Could you check a few things on this model? Use its own coordinates, in mm. A direction names the side the tool comes from. Give positions to 0.01 mm unless a question says otherwise; leave off trailing zeros. Order: outer loops, then holes, each group sorted by start corner. A loop starts at its lowest first (then second) coordinate and runs counter-clockwise, first axis right, second up. Notation, with made-up numbers: M -12,-4 L -7,-4 A20 cw -7,27 Z; hole C 77.5,59.25 d3. An arc over 180 degrees is marked long. Use a Markdown table: item, result. Add a question column.
Item 1: For faces 4 (the face through (-29.1, 13, -56)), 5 (the face through (-18, 13, -75)), 6 (the face through (-20.6, 3, 55)), 7 (the face through (-16, 3, -17)), which set-ups out of +Z, -Z, +X, -X, +Y, -Y let a thin tool reach every point of the face, with its end or its side?
Item 2: I'm going to push flat-ended pins straight in: pin 1 Ø3 at (x, z) = (0.5, -11.5) entering from +Y; pin 2 Ø2.5 at (y, z) = (10.94, -59.97) entering from +X; pin 3 Ø2 at (y, z) = (10.94, -59.97) entering from -X; pin 4 Ø8 at (y, z) = (6.87, -56.65) entering from -X. Where does each tip first touch, or does it pass through?
Item 3: If I drill on L1, parallel to Z at x = 13, y = 22.25; L2, parallel to Z at x = 23.5, y = 10.94; L3, parallel to Y at x = -11.5, z = -59.97, over which ranges is the centre line in solid material (lowest first)? Write a range as from..to.
Item 4: If we mould it in two halves opening along Y, with no side actions, what happens to faces 1 (the face through (16, 5.842, -61)), 2 (the face through (-15, 1.75, -69)), 3 (the face through (-2.3, 13, -69))? For each: released by +Y, released by -Y, zero draft, split by the parting line, or undercut.
Item 5: Suppose I cut it at C-C on y = 16. Write out the boundary of the cut face in (x, z).
Item 6: Suppose I cut it at D-D on z = -7. Write out the boundary of the cut face in (x, y).
Item 7: Suppose I cut it at A-A on x = -7.5. Write out the boundary of the cut face in (y, z) (3 decimals), plus the area to 3 significant figures.
Item 8: Suppose I cut it at B-B on z = -38. Write out the boundary of the cut face in (x, y).
from build123d import *

# Parameters (mm, degrees)
SKETCH1_W            = 66.8
SKETCH1_H            = 150
BOSS_EXTRUDE1_DEPTH  = 1.75
SKETCH2_W            = 7
SKETCH2_H            = 12
SKETCH2_W_2          = 2.3
BOSS_EXTRUDE2_DEPTH  = 6
SKETCH3_W            = 19
SKETCH3_H            = 5
BOSS_EXTRUDE3_DEPTH  = 11.79
SKETCH4_R            = 1.1
CUT_EXTRUDE1_DEPTH   = 23.3
SKETCH33_R           = 1.1
BOSS_EXTRUDE21_DEPTH = 1.5
SKETCH8_R            = 8.5
CUT_EXTRUDE3_DEPTH   = 4.3
SKETCH5_W            = 7
SKETCH5_H            = 7.697712298
CUT_EXTRUDE4_DEPTH   = 5
BOSS_EXTRUDE6_DEPTH  = 5
BOSS_EXTRUDE23_DEPTH = 4.3
CUT_EXTRUDE6_REACH   = 92.003
SKETCH36_R           = 3
SKETCH34_W           = 10
SKETCH34_H           = 5
BOSS_EXTRUDE24_DEPTH = 10.61
BOSS_EXTRUDE25_DEPTH = 4.3
BOSS_EXTRUDE26_DEPTH = 5
FILLET7_R            = 1
SKETCH44_W           = 5
SKETCH44_H           = 10.61
BOSS_EXTRUDE30_DEPTH = 14
SKETCH45_W           = 7
SKETCH45_H           = 0.4
CUT_EXTRUDE8_DEPTH   = 5
FILLET7_OF_MIRROR5_R = 1
SKETCH30_R           = 1.1
BOSS_EXTRUDE19_DEPTH = 0.6
SKETCH28_W           = 4.6
SKETCH28_H           = 12
BOSS_EXTRUDE31_DEPTH = 16.4
SKETCH47_W           = 66.8
SKETCH47_H           = 25.9
BOSS_EXTRUDE32_DEPTH = 1.5
SKETCH50_W           = 1.227389953
SKETCH50_H           = 22.4
BOSS_EXTRUDE33_DEPTH = 10.2
CUT_EXTRUDE9_DEPTH   = 2
SKETCH52_W           = 34
SKETCH52_H           = 53
SKETCH52_W_2         = 53
SKETCH52_H_2         = 34
BOSS_EXTRUDE34_DEPTH = 5.7
SKETCH53_W           = 26.2
SKETCH53_H           = 49.2
BOSS_EXTRUDE35_DEPTH = 2.8


# Read off the part's stored shape, not the designer's step: Boss-Extrude6
with BuildPart() as part:
    # Sketch1 → Boss-Extrude1 (new, symmetric)
    with BuildSketch(Plane(origin=(0, 0, 0), x_dir=(1, 0, 0), z_dir=(0, 1, 0))):
        Rectangle(SKETCH1_W, SKETCH1_H)
    boss_extrude1 = extrude(amount=BOSS_EXTRUDE1_DEPTH, both=True)

    # Sketch2 → Boss-Extrude2 (add)
    with BuildSketch(Plane(origin=(0, 1.75, 0), x_dir=(1, 0, 0), z_dir=(0, 1, 0))):
        with Locations((-29.9, 69)):
            Rectangle(SKETCH2_W, SKETCH2_H)
        with Locations((-1.15, 69)):
            Rectangle(SKETCH2_W_2, SKETCH2_H)
    boss_extrude2 = extrude(amount=BOSS_EXTRUDE2_DEPTH)

    # Sketch3 → Boss-Extrude3 (add)
    with BuildSketch(Plane(origin=(0, 1.75, 0), x_dir=(1, 0, 0), z_dir=(0, 1, 0))):
        with Locations((-19.6, 60.5)):
            Rectangle(SKETCH3_W, SKETCH3_H)
    boss_extrude3 = extrude(amount=BOSS_EXTRUDE3_DEPTH)

    # Sketch4 → Cut-Extrude1 (cut)
    with BuildSketch(Plane.ZY.offset(33.4)):
        with Locations((-59.97, 10.94)):
            Circle(SKETCH4_R)
    cut_extrude1 = extrude(amount=-CUT_EXTRUDE1_DEPTH, mode=Mode.SUBTRACT)

    # Sketch33 → Boss-Extrude21 (add)
    with BuildSketch(Plane.ZY.offset(29.1)):
        with BuildLine():
            Line((-58, 1.75), (-32.714619908, 1.75))
            Line((-32.714619908, 1.75), (-32.714619908, 18.755533204))
            ThreePointArc((-32.714619908, 18.755533204), (-32.928979134, 21.486214993), (-33.566805397, 24.15))
            Line((-33.566805397, 24.15), (-58, 24.15))
            Line((-58, 24.15), (-58, 1.75))
        make_face()
        with Locations((-50.214619908, 18.755533204)):
            Circle(SKETCH33_R, mode=Mode.SUBTRACT)
    boss_extrude21 = extrude(amount=-BOSS_EXTRUDE21_DEPTH)

    # Sketch8 → Cut-Extrude3 (cut)
    with BuildSketch(Plane.ZY.offset(29.1)):
        with Locations((-59.97, 10.94)):
            Circle(SKETCH8_R)
    cut_extrude3 = extrude(amount=CUT_EXTRUDE3_DEPTH, mode=Mode.SUBTRACT)

    # Sketch5 → Cut-Extrude4 (cut)
    with BuildSketch(Plane.XY.offset(-58)):
        with Locations((-15.6, 9.691143851)):
            Rectangle(SKETCH5_W, SKETCH5_H)
    cut_extrude4 = extrude(amount=-CUT_EXTRUDE4_DEPTH, mode=Mode.SUBTRACT)

    # Boss-Extrude6 outline → Boss-Extrude6 (add)
    with BuildSketch(Plane(origin=(-10.1, 0, 0), x_dir=(0, 0, -1), z_dir=(1, 0, 0))):
        with BuildLine():
            Line((63, 1.75), (63, 13.54))
            Line((63, 13.54), (58, 13.54))
            Line((58, 13.54), (54.474415859, 12.063241708))
            ThreePointArc((54.474415859, 12.063241708), (51.964403757, 9.99079907), (51.022610047, 6.875))
            Line((51.022610047, 6.875), (51.022610047, 1.75))
            Line((51.022610047, 1.75), (56.647610047, 1.75))
            ThreePointArc((56.647610047, 1.75), (55.965342342, 11.954383405), (58, 1.93165433))
            Line((58, 1.93165433), (58, 1.75))
            Line((58, 1.75), (63, 1.75))
        make_face()
    boss_extrude6 = extrude(amount=BOSS_EXTRUDE6_DEPTH)

    # Sketch35 → Boss-Extrude23 (add)
    with BuildSketch(Plane.ZY.offset(29.1)):
        with BuildLine():
            ThreePointArc((-51.696668378, 12.889867655), (-54.372371702, 4.543394851), (-63, 2.998394369))
            Line((-63, 2.998394369), (-63, 1.75))
            Line((-63, 1.75), (-32.714619908, 1.75))
            Line((-32.714619908, 1.75), (-32.714619908, 18.755533204))
            ThreePointArc((-32.714619908, 18.755533204), (-32.928979134, 21.486214993), (-33.566805397, 24.15))
            Line((-33.566805397, 24.15), (-47.475600378, 24.15))
            ThreePointArc((-47.475600378, 24.15), (-44.549583353, 16.631889912), (-51.696668378, 12.889867655))
        make_face()
        with BuildLine():
            ThreePointArc((-58, 19.208560939), (-57.114293593, 18.945931608), (-56.262320095, 18.588732556))
            ThreePointArc((-56.262320095, 18.588732556), (-55.413998212, 21.848907617), (-52.953639439, 24.15))
            Line((-52.953639439, 24.15), (-58, 24.15))
            Line((-58, 24.15), (-58, 19.208560939))
        make_face()
    boss_extrude23 = extrude(amount=BOSS_EXTRUDE23_DEPTH)

    # Cut-Extrude6: up to this face of the body (flat: up to its plane)
    cut_extrude6_end = Plane(part.part.faces().sort_by_distance((-19.1, 9.554283394, -60.558081983))[0])
    # Sketch36 → Cut-Extrude6 (cut, up to the picked face)
    with BuildSketch(Plane.ZY.offset(10.1), mode=Mode.PRIVATE) as cut_extrude6_sk1:
        with Locations((-56.647610047, 6.875)):
            Circle(SKETCH36_R)
    cut_extrude6_tool1 = split(extrude(cut_extrude6_sk1.sketch, amount=CUT_EXTRUDE6_REACH, mode=Mode.PRIVATE), bisect_by=cut_extrude6_end, keep=Keep.BOTH, mode=Mode.PRIVATE)
    cut_extrude6 = cut_extrude6_tool1.solids().sort_by(Axis((-10.1, 6.875, -56.64761), (-1, 0, 0)))[0]
    add(cut_extrude6, mode=Mode.SUBTRACT)

    # Sketch34 → Boss-Extrude24 (add)
    with BuildSketch(Plane(origin=(0, 13.54, 0), x_dir=(1, 0, 0), z_dir=(0, 1, 0))):
        with Locations((-24.1, 60.5)):
            Rectangle(SKETCH34_W, SKETCH34_H)
    boss_extrude24 = extrude(amount=BOSS_EXTRUDE24_DEPTH)

    # Sketch37 → Boss-Extrude25 (add)
    with BuildSketch(Plane.ZY.offset(29.1)):
        with BuildLine():
            Line((-58, 24.15), (-63, 24.15))
            Line((-63, 24.15), (-63, 18.881605631))
            ThreePointArc((-63, 18.881605631), (-60.524639471, 19.421885112), (-58, 19.208560939))
            Line((-58, 19.208560939), (-58, 24.15))
        make_face()
    boss_extrude25 = extrude(amount=BOSS_EXTRUDE25_DEPTH)

    # Sketch38 → Boss-Extrude26 (add)
    with BuildSketch(Plane.ZY.offset(10.1)):
        with BuildLine():
            Line((-56.647610047, 1.75), (-58.2, 1.75))
            Line((-58.2, 1.75), (-58.2, 1.99076921))
            ThreePointArc((-58.2, 1.99076921), (-57.433085123, 1.810549991), (-56.647610047, 1.75))
        make_face()
    boss_extrude26 = extrude(amount=-BOSS_EXTRUDE26_DEPTH)

    # Fillet7
    fillet7_edges = [part.edges().sort_by_distance(p)[0] for p in [
        (-31.25, 12.889867655, -51.696668378),
        (-31.25, 24.15, -47.475600378),
        (-31.25, 18.588732556, -56.262320095),
        (-31.25, 24.15, -52.953639439),
        (-11.1, 9.552880023, -58),
        (-33.4, 7.75, -71.424349566),
        (-27.75, 7.75, -63),
        (-27.6, 12.95, -58),
    ]]
    fillet(fillet7_edges, radius=FILLET7_R)

    # Sketch44 → Boss-Extrude30 (add)
    with BuildSketch(Plane(origin=(-19.1, 0, 0), x_dir=(0, 0, -1), z_dir=(1, 0, 0))):
        with Locations((60.5, 18.845)):
            Rectangle(SKETCH44_W, SKETCH44_H)
    boss_extrude30 = extrude(amount=BOSS_EXTRUDE30_DEPTH)

    # Sketch45 → Cut-Extrude8 (cut)
    with BuildSketch(Plane.XY.offset(-58)):
        with Locations((-15.6, 13.74)):
            Rectangle(SKETCH45_W, SKETCH45_H)
    cut_extrude8 = extrude(amount=-CUT_EXTRUDE8_DEPTH, mode=Mode.SUBTRACT)

    # Mirror5: Boss-Extrude1, Boss-Extrude2, Boss-Extrude3, Cut-Extrude1, Boss-Extrude21, Cut-Extrude3, Cut-Extrude4, Boss-Extrude6, Boss-Extrude23, Cut-Extrude6, Boss-Extrude24, Boss-Extrude25, Boss-Extrude26, Boss-Extrude30, Cut-Extrude8 across plane
    add(boss_extrude1.mirror(Plane(origin=(0, 0, 0), x_dir=(0, 0, 1), z_dir=(1, 0, 0))))
    add(boss_extrude2.mirror(Plane(origin=(0, 0, 0), x_dir=(0, 0, 1), z_dir=(1, 0, 0))))
    add(boss_extrude3.mirror(Plane(origin=(0, 0, 0), x_dir=(0, 0, 1), z_dir=(1, 0, 0))))
    add(cut_extrude1.mirror(Plane(origin=(0, 0, 0), x_dir=(0, 0, 1), z_dir=(1, 0, 0))), mode=Mode.SUBTRACT)
    add(boss_extrude21.mirror(Plane(origin=(0, 0, 0), x_dir=(0, 0, 1), z_dir=(1, 0, 0))))
    add(cut_extrude3.mirror(Plane(origin=(0, 0, 0), x_dir=(0, 0, 1), z_dir=(1, 0, 0))), mode=Mode.SUBTRACT)
    add(cut_extrude4.mirror(Plane(origin=(0, 0, 0), x_dir=(0, 0, 1), z_dir=(1, 0, 0))), mode=Mode.SUBTRACT)
    add(boss_extrude6.mirror(Plane(origin=(0, 0, 0), x_dir=(0, 0, 1), z_dir=(1, 0, 0))))
    add(boss_extrude23.mirror(Plane(origin=(0, 0, 0), x_dir=(0, 0, 1), z_dir=(1, 0, 0))))
    add(cut_extrude6.mirror(Plane(origin=(0, 0, 0), x_dir=(0, 0, 1), z_dir=(1, 0, 0))), mode=Mode.SUBTRACT)
    add(boss_extrude24.mirror(Plane(origin=(0, 0, 0), x_dir=(0, 0, 1), z_dir=(1, 0, 0))))
    add(boss_extrude25.mirror(Plane(origin=(0, 0, 0), x_dir=(0, 0, 1), z_dir=(1, 0, 0))))
    add(boss_extrude26.mirror(Plane(origin=(0, 0, 0), x_dir=(0, 0, 1), z_dir=(1, 0, 0))))
    add(boss_extrude30.mirror(Plane(origin=(0, 0, 0), x_dir=(0, 0, 1), z_dir=(1, 0, 0))))
    add(cut_extrude8.mirror(Plane(origin=(0, 0, 0), x_dir=(0, 0, 1), z_dir=(1, 0, 0))), mode=Mode.SUBTRACT)

    # Fillet7 of Mirror5
    fillet7_of_mirror5_edges = [part.edges().sort_by_distance(p)[0] for p in [
        (31.25, 12.889867655, -51.696668378),
        (31.25, 24.15, -47.475600378),
        (31.25, 18.588732556, -56.262320095),
        (31.25, 24.15, -52.953639439),
        (11.1, 9.552880023, -58),
        (33.4, 7.75, -71.424349566),
        (27.75, 7.75, -63),
        (27.6, 12.95, -58),
    ]]
    fillet(fillet7_of_mirror5_edges, radius=FILLET7_OF_MIRROR5_R)

    # Sketch30 → Boss-Extrude19 (add)
    with BuildSketch(Plane(origin=(-10.1, 0, 0), x_dir=(0, 0, -1), z_dir=(1, 0, 0))):
        with Locations(Location((59.97, 10.94, 0), (0, 0, 90))):
            Circle(SKETCH30_R)
    boss_extrude19 = extrude(amount=-BOSS_EXTRUDE19_DEPTH)

    # Mirror6: Boss-Extrude19 across plane
    add(boss_extrude19.mirror(Plane(origin=(0, 0, 0), x_dir=(0, 0, 1), z_dir=(1, 0, 0))))

    # Sketch28 → Boss-Extrude31 (add)
    with BuildSketch(Plane(origin=(0, 7.75, 0), x_dir=(1, 0, 0), z_dir=(0, 1, 0))):
        with Locations((0, 69)):
            Rectangle(SKETCH28_W, SKETCH28_H)
    extrude(amount=BOSS_EXTRUDE31_DEPTH)

    # Sketch47 → Boss-Extrude32 (add)
    with BuildSketch(Plane(origin=(0, 0, -75), x_dir=(-1, 0, 0), z_dir=(0, 0, -1))):
        with Locations((0, 11.2)):
            Rectangle(SKETCH47_W, SKETCH47_H)
    extrude(amount=BOSS_EXTRUDE32_DEPTH)

    # Sketch50 → Boss-Extrude33 (add)
    with BuildSketch(Plane.ZY.offset(-5.1)):
        with Locations((-62.386305024, 12.95)):
            Rectangle(SKETCH50_W, SKETCH50_H)
    extrude(amount=BOSS_EXTRUDE33_DEPTH)

    # Sketch51 → Cut-Extrude9 (cut)
    with BuildSketch(Plane(origin=(0, 1.75, 0), x_dir=(1, 0, 0), z_dir=(0, 1, 0))):
        with BuildLine():
            Line((-33.4, 32.714619908), (-33.4, -75))
            Line((-33.4, -75), (33.4, -75))
            Line((33.4, -75), (33.4, 32.714619908))
            Line((33.4, 32.714619908), (27.6, 32.714619908))
            Line((27.6, 32.714619908), (27.6, 57))
            ThreePointArc((27.6, 57), (27.307106781, 57.707106781), (26.6, 58))
            Line((26.6, 58), (10.1, 58))
            Line((10.1, 58), (10.1, 56.647610047))
            Line((10.1, 56.647610047), (10.1, 51.022610047))
            Line((10.1, 51.022610047), (5.1, 51.022610047))
            Line((5.1, 51.022610047), (5.1, 56.647610047))
            Line((5.1, 56.647610047), (5.1, 61.772610047))
            Line((5.1, 61.772610047), (-5.1, 61.772610047))
            Line((-5.1, 61.772610047), (-5.1, 56.647610047))
            Line((-5.1, 56.647610047), (-5.1, 51.022610047))
            Line((-5.1, 51.022610047), (-10.1, 51.022610047))
            Line((-10.1, 51.022610047), (-10.1, 56.647610047))
            Line((-10.1, 56.647610047), (-10.1, 58))
            Line((-10.1, 58), (-26.6, 58))
            ThreePointArc((-26.6, 58), (-27.307106781, 57.707106781), (-27.6, 57))
            Line((-27.6, 57), (-27.6, 32.714619908))
            Line((-27.6, 32.714619908), (-33.4, 32.714619908))
        make_face()
    extrude(amount=-CUT_EXTRUDE9_DEPTH, mode=Mode.SUBTRACT)

    # Sketch52 → Boss-Extrude34 (add)
    with BuildSketch(Plane(origin=(0, -0.25, 0), x_dir=(1, 0, 0), z_dir=(0, 1, 0))):
        with Locations((-15.4, -9.5)):
            Rectangle(SKETCH52_W, SKETCH52_H)
        with Locations((5.9, -55)):
            Rectangle(SKETCH52_W_2, SKETCH52_H_2)
    extrude(amount=BOSS_EXTRUDE34_DEPTH)

    # Sketch53 → Boss-Extrude35 (add)
    with BuildSketch(Plane(origin=(0, -0.25, 0), x_dir=(1, 0, 0), z_dir=(0, 1, 0))):
        with Locations((19.3, -12.4)):
            Rectangle(SKETCH53_W, SKETCH53_H)
    extrude(amount=BOSS_EXTRUDE35_DEPTH)


solid = part.part
Findings below:
| question | item | result |
|---|---|---|
| 1 | face 4 | -X |
| 1 | face 5 | +Y |
| 1 | face 6 | +Z, -X, +Y |
| 1 | face 7 | +X, -X, +Y |
| 2 | pin 1 | stops at y = 5.45 |
| 2 | pin 2 | stops at x = 29.1 |
| 2 | pin 3 | stops at x = -10.7 |
| 2 | pin 4 | stops at x = -33.4 |
| 3 | L1 | z = -76.5..-75, -63..-58 |
| 3 | L2 | z = -76.5..-75, -63..-61.07, -58.87..-58 |
| 3 | L3 | y = -1.75..9.84, 12.04..24.15 |
| 4 | face 1 | undercut |
| 4 | face 2 | released by +Y |
| 4 | face 3 | zero draft |
| 5 | outline | M -33.4,-76.5 L 33.4,-76.5 L 33.4,-75 L 2.3,-75 L 2.3,-63 L 29.1,-63 L 29.1,-44.83 L 33.4,-44.83 L 33.4,-32.71 L 27.6,-32.71 L 27.6,-57 A1 cw 26.6,-58 L 5.1,-58 L 5.1,-61.77 L -5.1,-61.77 L -5.1,-58 L -26.6,-58 A1 cw -27.6,-57 L -27.6,-32.71 L -33.4,-32.71 L -33.4,-44.83 L -29.1,-44.83 L -29.1,-63 L -2.3,-63 L -2.3,-75 L -33.4,-75 Z |
| 6 | outline | M -33.4,-1.75 L 33.4,-1.75 L 33.4,-0.25 L 32.4,-0.25 L 32.4,2.55 L 6.2,2.55 L 6.2,-0.25 L 1.6,-0.25 L 1.6,5.45 L -32.4,5.45 L -32.4,-0.25 L -33.4,-0.25 Z |
| 7 | outline | M -1.75,-76.5 L 24.15,-76.5 L 24.15,-75 L 1.75,-75 L 1.75,-63 L 24.15,-63 L 24.15,-58 L 13.54,-58 L 12.063,-54.474 A5.625 ccw 6.875,-51.023 L -0.25,-51.023 L -0.25,-17 L 5.45,-17 L 5.45,36 L -0.25,36 L -0.25,38 L 5.45,38 L 5.45,72 L -0.25,72 L -0.25,75 L -1.75,75 Z; hole C 6.875,-56.648 d10.25 |
| 7 | area | 907 mm^2 |
| 8 | outline | M -33.4,-1.75 L 33.4,-1.75 L 33.4,24.15 L 27.6,24.15 L 27.6,-0.25 L -27.6,-0.25 L -27.6,24.15 L -33.4,24.15 Z |
